Autodesk Inventor part; units mm, degrees
ref_plane "Work Plane1" through (0, 0, 0) normal (0, 0, 1) x (1, 0, 0)
ref_plane "YZ Plane" through (0, 0, 0) normal (1, 0, 0) x (0, 1, 0)
ref_plane "XZ Plane" through (0, 0, 0) normal (0, 1, 0) x (-1, 0, 0)
sketch "Sketch1" plane through (0, 0, 0) normal (0, 0, 1) x (1, 0, 0)
  line L0 (0.1212, -19.5) -> (-0.3333, -19.5)
  line L1 (0.1212, -20) -> (0.1212, -19.5)
  line L2 (5.1624, -20) -> (0.1212, -20)
  arc A0 (5.1624, -20) -> (6.6667, -18.4957) centre (5.1624, -18.4957) ccw
  line L3 (6.6667, -13.3333) -> (6.6667, -18.4957)
  line L4 (6.2121, -13.3333) -> (6.6667, -13.3333)
  line L5 (6.2121, -13) -> (6.2121, -13.3333)
  line L6 (5.0758, -13) -> (6.2121, -13)
  line L7 (5.0758, -16) -> (5.0758, -13)
  line L8 (3.7121, -16) -> (5.0758, -16)
  line L9 (1.2121, -13.3333) -> (3.7121, -16)
  line L10 (1.2121, -10.8302) -> (1.2121, -13.3333)
  arc A1 (1.2121, -9.1698) -> (1.2121, -10.8302) centre (1.483, -10) ccw
  line L11 (1.2121, -6.5455) -> (1.2121, -9.1698)
  line L12 (3.6667, -4.0909) -> (1.2121, -6.5455)
  line L13 (5.1667, -4.0909) -> (3.6667, -4.0909)
  line L14 (5.1667, -7) -> (5.1667, -4.0909)
  line L15 (6.1667, -7) -> (5.1667, -7)
  line L16 (6.1667, -6.5455) -> (6.1667, -7)
  line L17 (6.6667, -6.5455) -> (6.1667, -6.5455)
  line L18 (6.6667, -1.5043) -> (6.6667, -6.5455)
  arc A2 (6.6667, -1.5043) -> (5.1624, 0) centre (5.1624, -1.5043) ccw
  line L19 (0, 0) -> (5.1624, 0)
  line L20 (0, -0.4545) -> (0, 0)
  line L21 (-0.3333, -0.4545) -> (0, -0.4545)
  line L22 (-0.3333, -1.5909) -> (-0.3333, -0.4545)
  line L23 (2.6667, -1.5909) -> (-0.3333, -1.5909)
  line L24 (2.6667, -2.9545) -> (2.6667, -1.5909)
  line L25 (0, -5.4545) -> (2.6667, -2.9545)
  line L26 (-2.5032, -5.4545) -> (0, -5.4545)
  arc A3 (-4.1635, -5.4545) -> (-2.5032, -5.4545) centre (-3.3333, -5.1837) ccw
  line L27 (-6.7879, -5.4545) -> (-4.1635, -5.4545)
  line L28 (-9.2424, -3) -> (-6.7879, -5.4545)
  line L29 (-9.2424, -1.5) -> (-9.2424, -3)
  line L30 (-6.3333, -1.5) -> (-9.2424, -1.5)
  line L31 (-6.3333, -0.5) -> (-6.3333, -1.5)
  line L32 (-6.7879, -0.5) -> (-6.3333, -0.5)
  line L33 (-6.7879, 0) -> (-6.7879, -0.5)
  line L34 (-11.829, 0) -> (-6.7879, 0)
  arc A4 (-11.829, 0) -> (-13.3333, -1.5043) centre (-11.829, -1.5043) ccw
  line L35 (-13.3333, -6.6667) -> (-13.3333, -1.5043)
  line L36 (-12.8788, -6.6667) -> (-13.3333, -6.6667)
  line L37 (-12.8788, -7) -> (-12.8788, -6.6667)
  line L38 (-11.7424, -7) -> (-12.8788, -7)
  line L39 (-11.7424, -4) -> (-11.7424, -7)
  line L40 (-10.3788, -4) -> (-11.7424, -4)
  line L41 (-7.8788, -6.6667) -> (-10.3788, -4)
  line L42 (-7.8788, -9.1698) -> (-7.8788, -6.6667)
  arc A5 (-7.8788, -10.8302) -> (-7.8788, -9.1698) centre (-8.1497, -10) ccw
  line L43 (-7.8788, -13.4545) -> (-7.8788, -10.8302)
  line L44 (-10.3333, -15.9091) -> (-7.8788, -13.4545)
  line L45 (-11.8333, -15.9091) -> (-10.3333, -15.9091)
  line L46 (-11.8333, -13) -> (-11.8333, -15.9091)
  line L47 (-12.8333, -13) -> (-11.8333, -13)
  line L48 (-12.8333, -13.4545) -> (-12.8333, -13)
  line L49 (-13.3333, -13.4545) -> (-12.8333, -13.4545)
  line L50 (-13.3333, -18.4957) -> (-13.3333, -13.4545)
  arc A6 (-13.3333, -18.4957) -> (-11.829, -20) centre (-11.829, -18.4957) ccw
  line L51 (-6.6667, -20) -> (-11.829, -20)
  line L52 (-6.6667, -19.5455) -> (-6.6667, -20)
  line L53 (-6.3333, -19.5455) -> (-6.6667, -19.5455)
  line L54 (-6.3333, -18.4091) -> (-6.3333, -19.5455)
  line L55 (-9.3333, -18.4091) -> (-6.3333, -18.4091)
  line L56 (-9.3333, -17.0455) -> (-9.3333, -18.4091)
  line L57 (-6.6667, -14.5455) -> (-9.3333, -17.0455)
  line L58 (-4.1635, -14.5455) -> (-6.6667, -14.5455)
  arc A7 (-2.5032, -14.5455) -> (-4.1635, -14.5455) centre (-3.3333, -14.8163) ccw
  line L59 (0.1212, -14.5455) -> (-2.5032, -14.5455)
  line L60 (2.5758, -17) -> (0.1212, -14.5455)
  line L61 (2.5758, -18.5) -> (2.5758, -17)
  line L62 (-0.3333, -18.5) -> (2.5758, -18.5)
  line L63 (-0.3333, -19.5) -> (-0.3333, -18.5)
  line L64 (-1.523, -12.9923) -> (-2.0717, -12.4435)
  arc A8 (-4.5949, -12.4435) -> (-2.0717, -12.4435) centre (-3.3333, -10) ccw
  line L65 (-4.5949, -12.4435) -> (-5.1437, -12.9923)
  line L66 (-5.1437, -12.9923) -> (-6.3256, -11.8104)
  line L67 (-6.3256, -11.8104) -> (-5.7769, -11.2616)
  arc A9 (-5.7769, -8.7384) -> (-5.7769, -11.2616) centre (-3.3333, -10) ccw
  line L68 (-5.7769, -8.7384) -> (-6.3256, -8.1896)
  line L69 (-6.3256, -8.1896) -> (-5.1437, -7.0077)
  line L70 (-5.1437, -7.0077) -> (-4.5949, -7.5565)
  arc A10 (-2.0717, -7.5565) -> (-4.5949, -7.5565) centre (-3.3333, -10) ccw
  line L71 (-2.0717, -7.5565) -> (-1.523, -7.0077)
  line L72 (-1.523, -7.0077) -> (-0.3411, -8.1896)
  line L73 (-0.3411, -8.1896) -> (-0.8898, -8.7384)
  arc A11 (-0.8898, -11.2616) -> (-0.8898, -8.7384) centre (-3.3333, -10) ccw
  line L74 (-0.8898, -11.2616) -> (-0.3411, -11.8104)
  line L75 (-0.3411, -11.8104) -> (-1.523, -12.9923)
  point P0 (-13.3333, -20)
extrude "Extrusion1" add sketch "Sketch1" along normal mid plane 165.1
ref_plane "Work Plane1" through (0, 0, 0) normal (0, 0, 1) x (1, 0, 0)
properties part number "Lift Connector"
Design review of the part built by this model. Coordinates are the model's own, in mm. A direction names the side the tool comes from. Coordinates: 2 decimals unless noted, no trailing zeros. Answer as a JSON object with one key per item and string values.
Item 1: Insertion check: pin 1 Ø0.8 at (x, z) = (-5, 29) entering from +Y; pin 2 Ø0.5 at (x, z) = (-13, 38.5) entering from -Y; pin 3 Ø1.2 at (x, z) = (6, -31.5) entering from +Y. Each pin has a flat end and moves straight along its axis. Give the tip position at first contact, or say it passes through.
Outcome:
{"pin 1": "y = -5.45", "pin 2": "y = -19.69", "pin 3": "y = -0.02"}
Item 2: Machinability: for faces 3 (the flat face through (1, -12, -82.55)), 4 (the flat face through (1.212, -8, -1)), which of the approach directions +Z, -Z, +X, -X, +Y, -Y give a long, thin tool a straight path to every point of the face, cutting with its end or side? Answer none if there is none.
Outcome:
{"face 3": "-Z, +X, -X, +Y, -Y", "face 4": "+Z, -Z"}
Item 3: Wall thickness on probe 1 along Y at (x, z) = (5, -67); probe 2 along X at (y, z) = (-14.25, 2.5); probe 3 along X at (y, z) = (-2, -15.5): over which ranges is each line inside the solid? List them lowest first.
Outcome:
{"probe 1": "-20 to -16, -4.09 to 0", "probe 2": "-13.33 to -11.83, -8.67 to -4, -2.67 to 2.07, 5.08 to 6.67", "probe 3": "-13.33 to -9.24, 2.67 to 6.67"}
Item 4: Draft analysis for pull direction Y (two halves, no side actions). For faces 1 (the flat face through (6.667, -4, -1)), 2 (the flat face through (-7.879, -12, -1)), state which applies: pulls with the +Y half, pulls with the -Y half, needs draft (parallel to the pull), parting line crosses it, or undercut.
Outcome:
{"face 1": "needs draft", "face 2": "undercut"}
